Geometry: final body of the model. Coordinates: model frame, mm. A direction names the side the tool comes from. Round coordinates to 2 decimals unless told otherwise and drop trailing zeros. Order: outer loops, then holes, each group sorted by start corner. A loop starts at its lowest first (then second) coordinate and runs counter-clockwise, first axis right, second up. Notation, with made-up numbers: (68.5, -18.75) -> (94.5, -18.75) arc R29 ccw to (94.5, 16.25) -> close; hole circle Ø3 at (36.5, -24). An arc over 180 degrees is marked (long way). Put each result on its own line as item: value.
```python
from build123d import *

# Parameters (mm, degrees)
SKETCH_2_W          = 42.3
SKETCH_2_H          = 42.3
EXTRUDE_1_DEPTH     = 28
SKETCH_3_R          = 11
EXTRUDE_2_DEPTH     = 2
EXTRUDE_START       = -2
SKETCH_4_R          = 2.5
EXTRUDE_3_DEPTH     = 24
SKETCH_5_R          = 1.5
CUT_EXTRUDE_1_DEPTH = 4.5
CHAMFER_1_SIZE      = 4
CUT_EXTRUDE_START   = -8
SKETCH_6_OUTSIDE_W  = 60.152
SKETCH_6_OUTSIDE_H  = 60.152
CUT_EXTRUDE_2_DEPTH = 12
SKETCH_7_R          = 2.5
EXTRUDE_4_DEPTH     = 2
CHAMFER_2_SIZE      = 1
SKETCH_8_W          = 14
SKETCH_8_H          = 5
EXTRUDE_5_DEPTH     = 6


with BuildPart() as part:
    # Эскиз2 → Бобышка-Вытянуть1 (new body)
    with BuildSketch(Plane(origin=(0, 0, 0), x_dir=(1, 0, 0), z_dir=(0, 1, 0))):
        Rectangle(SKETCH_2_W, SKETCH_2_H)
    extrude(amount=EXTRUDE_1_DEPTH)

    # Эскиз3 → Бобышка-Вытянуть2 (add)
    with BuildSketch(Plane(origin=(0, 28, 0), x_dir=(1, 0, 0), z_dir=(0, 1, 0))):
        Circle(SKETCH_3_R)
    extrude(amount=EXTRUDE_2_DEPTH)

    # Эскиз4 → Бобышка-Вытянуть3 (add)
    with BuildSketch(Plane(origin=(0, 30, 0), x_dir=(1, 0, 0), z_dir=(0, 1, 0)).offset(EXTRUDE_START)):
        Circle(SKETCH_4_R)
    extrude(amount=EXTRUDE_3_DEPTH)

    # Эскиз5 → Вырез-Вытянуть1 (cut)
    with BuildSketch(Plane(origin=(0, 28, 0), x_dir=(1, 0, 0), z_dir=(0, 1, 0))):
        with Locations((-15.5, 15.5)):
            Circle(SKETCH_5_R)
        with Locations((15.5, 15.5)):
            Circle(SKETCH_5_R)
        with Locations((15.5, -15.5)):
            Circle(SKETCH_5_R)
        with Locations((-15.5, -15.5)):
            Circle(SKETCH_5_R)
    extrude(amount=-CUT_EXTRUDE_1_DEPTH, mode=Mode.SUBTRACT)

    # Фаска1
    chamfer_1_edges = [part.edges().sort_by_distance(p)[0] for p in [
        (21.15, 14, 21.15),
        (-21.15, 14, 21.15),
        (-21.15, 14, -21.15),
        (21.15, 14, -21.15),
    ]]
    chamfer(chamfer_1_edges, length=CHAMFER_1_SIZE)

    # Эскиз6 outside → Вырез-Вытянуть2 (cut)
    with BuildSketch(Plane(origin=(0, 28, 0), x_dir=(1, 0, 0), z_dir=(0, 1, 0)).offset(CUT_EXTRUDE_START)):
        Rectangle(SKETCH_6_OUTSIDE_W, SKETCH_6_OUTSIDE_H)
        Polygon((-20.75, 16.984314575), (-20.75, -16.984314575), (-16.984314575, -20.75), (16.984314575, -20.75), (20.75, -16.984314575), (20.75, 16.984314575), (16.984314575, 20.75), (-16.984314575, 20.75), align=None, mode=Mode.SUBTRACT)
    extrude(amount=-CUT_EXTRUDE_2_DEPTH, mode=Mode.SUBTRACT)

    # Эскиз7 → Бобышка-Вытянуть4 (add)
    with BuildSketch(Plane.XZ):
        with Locations((-15.5, -15.5)):
            Circle(SKETCH_7_R)
        with Locations((15.5, -15.5)):
            Circle(SKETCH_7_R)
        with Locations((15.5, 15.5)):
            Circle(SKETCH_7_R)
        with Locations((-15.5, 15.5)):
            Circle(SKETCH_7_R)
    extrude(amount=EXTRUDE_4_DEPTH)

    # Фаска2
    chamfer_2_edges = [part.edges().sort_by_distance(p)[0] for p in [
        (-18, -2, -15.5),
        (13, -2, -15.5),
        (13, -2, 15.5),
        (-18, -2, 15.5),
    ]]
    chamfer(chamfer_2_edges, length=CHAMFER_2_SIZE)

    # Эскиз8 → Бобышка-Вытянуть5 (add)
    with BuildSketch(Plane(origin=(21.15, 0, 0), x_dir=(0, 0, -1), z_dir=(1, 0, 0))):
        with Locations((0, 2.5)):
            Rectangle(SKETCH_8_W, SKETCH_8_H)
    extrude(amount=EXTRUDE_5_DEPTH)


solid = part.part
```
1. Cut plane A-A on y = 6. Return loops of the section in (x, z), and give its area (3 significant figures).
Ans:
outline: (-21.15, -17.15) -> (-17.15, -21.15) -> (17.15, -21.15) -> (21.15, -17.15) -> (21.15, 17.15) -> (17.15, 21.15) -> (-17.15, 21.15) -> (-21.15, 17.15) -> close
area: 1,760 mm²
2. Contact query for flat-ended pins moving along their axis: P1, Ø2.5, axis at x = -15, z = 16, coming from the +Y side; P2, Ø1, axis at x = 6.5, z = -5.5, coming from the -Y side; P3, Ø2.5, axis at x = 15.5, z = 15.5, coming from the +Y side. Output: stop coordinate, or through.
Ans:
P1: y = 28
P2: y = 0
P3: y = 23.5
3. Cut plane B-B on z = 0. Return loops of the section in (x, y), and give its area (3 significant figures).
Ans:
outline: (-21.15, 0) -> (27.15, 0) -> (27.15, 5) -> (21.15, 5) -> (21.15, 8) -> (20.75, 8) -> (20.75, 20) -> (21.15, 20) -> (21.15, 28) -> (11, 28) -> (11, 30) -> (2.5, 30) -> (2.5, 52) -> (-2.5, 52) -> (-2.5, 30) -> (-11, 30) -> (-11, 28) -> (-21.15, 28) -> (-21.15, 20) -> (-20.75, 20) -> (-20.75, 8) -> (-21.15, 8) -> close
area: 1,360 mm²
4. Draft query along X for faces 1 (the face through (19.2, 23.9, -19.1)), 2 (the face through (0, 24, -21.15)), 3 (the face through (-18.841, 14.084, -18.894)), 4 (the face through (-16, 23.5, -16)). Return one class per face: +X half, -X half, draft (parallel to the pull), parting line (faces both ways), or undercut.
Ans:
face 1: +X half
face 2: draft
face 3: -X half
face 4: undercut
5. Cut plane D-D on x = 12. Return loops of the section in (y, z), and give its area (3 significant figures).
Ans:
outline: (0, -21.15) -> (8, -21.15) -> (8, -20.75) -> (20, -20.75) -> (20, -21.15) -> (28, -21.15) -> (28, 21.15) -> (20, 21.15) -> (20, 20.75) -> (8, 20.75) -> (8, 21.15) -> (0, 21.15) -> close
area: 1,170 mm²
6. Set-up query: faces 5 (the face through (24, 2, 7)), 6 (the face through (14, 25.78, -15.57)), 7 (the face through (13, -0.5, 15.6)), 8 (the face through (-16, -2, -15)), 9 (the face through (-18.894, 14.084, 18.841)). Return all of +Z, -Z, +X, -X, +Y, -Y with unobstructed straight access to the full face (end or side cutting, diameter ignored); none if empty.
Ans:
face 5: +Z, +X, +Y, -Y
face 6: +Y
face 7: -Y
face 8: +Z, -Z, +X, -X, -Y
face 9: +Z, -X
7. Material intervals for probe 1 along Z at (x, y) = (15.5, 25); probe 2 along Z at (x, y) = (-15, 26), sorted ascending.
Ans:
probe 1: -21.15 to -17, -14 to 14, 17 to 21.15
probe 2: -21.15 to -16.91, -14.09 to 14.09, 16.91 to 21.15
8. Cut plane C-C on x = 0. Return loops of the section in (y, z).
Ans:
outline: (0, -21.15) -> (8, -21.15) -> (8, -20.75) -> (20, -20.75) -> (20, -21.15) -> (28, -21.15) -> (28, -11) -> (30, -11) -> (30, -2.5) -> (52, -2.5) -> (52, 2.5) -> (30, 2.5) -> (30, 11) -> (28, 11) -> (28, 21.15) -> (20, 21.15) -> (20, 20.75) -> (8, 20.75) -> (8, 21.15) -> (0, 21.15) -> close
